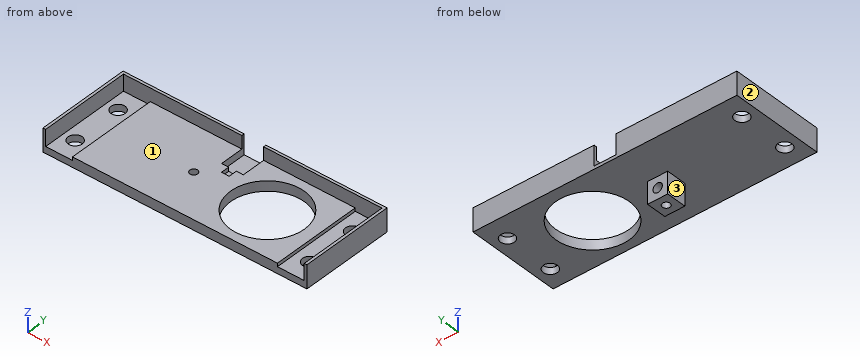
```python
from build123d import *

# Parameters (mm, degrees)
SKETCH_W        = 78.8
SKETCH_H        = 28
PAD_DEPTH       = 3
SKETCH001_R     = 11
POCKET_DEPTH    = 3.9
SKETCH002_W     = 0.8
SKETCH002_H     = 28
PAD001_DEPTH    = 3.9
SKETCH003_W     = 77.2
SKETCH003_H     = 0.8
PAD002_DEPTH    = 3.9
SKETCH004_W     = 8
SKETCH004_H     = 27.2
POCKET001_DEPTH = 1
SKETCH005_R     = 2.1
POCKET002_DEPTH = 5
SKETCH006_W     = 6
SKETCH006_H     = 6
PAD003_DEPTH    = 6.5
SKETCH007_R     = 1.15
POCKET003_DEPTH = 10
SKETCH008_R     = 1.4
POCKET004_DEPTH = 6
SKETCH009_W     = 2.3
SKETCH009_H     = 2.5
POCKET005_DEPTH = 1.2
SKETCH011_W     = 6.5
SKETCH011_H     = 8
POCKET006_DEPTH = 6


with BuildPart() as part:
    # Sketch → Pad (new body)
    with BuildSketch(Plane.XY):
        with Locations((0, 0.4)):
            Rectangle(SKETCH_W, SKETCH_H)
    extrude(amount=PAD_DEPTH)

    # Sketch001 (on Face6 of Pad) → Pocket (cut)
    with BuildSketch(Plane.XY.offset(3)):
        with Locations((16, 0)):
            Circle(SKETCH001_R)
    extrude(amount=-POCKET_DEPTH, mode=Mode.SUBTRACT)

    # Sketch002 (on Face5 of Pocket) → Pad001 (join)
    with BuildSketch(Plane.XY.offset(3)):
        with Locations((39, 0.4)):
            Rectangle(SKETCH002_W, SKETCH002_H)
        with Locations((-39, 0.4)):
            Rectangle(SKETCH002_W, SKETCH002_H)
    extrude(amount=PAD001_DEPTH)

    # Sketch003 (on Face6 of Pad001) → Pad002 (join)
    with BuildSketch(Plane.XY.offset(3)):
        with Locations((0, 14)):
            Rectangle(SKETCH003_W, SKETCH003_H)
    extrude(amount=PAD002_DEPTH)

    # Sketch004 (on Face16 of Pad002) → Pocket001 (cut)
    with BuildSketch(Plane.XY.offset(3)):
        with Locations((34.6, 0)):
            Rectangle(SKETCH004_W, SKETCH004_H)
        with Locations((-34.6, 0)):
            Rectangle(SKETCH004_W, SKETCH004_H)
    extrude(amount=-POCKET001_DEPTH, mode=Mode.SUBTRACT)

    # Sketch005 (on Face19 of Pocket001) → Pocket002 (cut)
    with BuildSketch(Plane.XY.offset(3)):
        with Locations((35, 7.5)):
            Circle(SKETCH005_R)
        with Locations((35, -7.5)):
            Circle(SKETCH005_R)
        with Locations((-35, 7.5)):
            Circle(SKETCH005_R)
        with Locations((-35, -7.5)):
            Circle(SKETCH005_R)
    extrude(amount=-POCKET002_DEPTH, mode=Mode.SUBTRACT)

    # Sketch006 (on Face4 of Pocket002) → Pad003 (join)
    with BuildSketch(Plane(origin=(0, 0, 0), x_dir=(1, 0, 0), z_dir=(0, 0, -1))):
        with Locations((-6, 0)):
            Rectangle(SKETCH006_W, SKETCH006_H)
    extrude(amount=PAD003_DEPTH)

    # Sketch007 (on Face32 of Pad003) → Pocket003 (cut)
    with BuildSketch(Plane(origin=(0, 0, -6.5), x_dir=(1, 0, 0), z_dir=(0, 0, -1))):
        with Locations((-6, 0)):
            Circle(SKETCH007_R)
    extrude(amount=-POCKET003_DEPTH, mode=Mode.SUBTRACT)

    # Sketch008 (on Face15 of Pocket003) → Pocket004 (cut)
    with BuildSketch(Plane.XZ.offset(3)):
        with Locations((-6, -3.25)):
            Circle(SKETCH008_R)
    extrude(amount=-POCKET004_DEPTH, mode=Mode.SUBTRACT)

    # Sketch009 (on Face27 of Pocket004) → Pocket005 (cut)
    with BuildSketch(Plane.XY.offset(3)):
        with Locations((0, 5.25)):
            Rectangle(SKETCH009_W, SKETCH009_H)
    extrude(amount=-POCKET005_DEPTH, mode=Mode.SUBTRACT)

    # Sketch011 (on Face21 of Pocket005) → Pocket006 (cut)
    with BuildSketch(Plane.XY.offset(6.9)):
        with Locations((0, 10.5)):
            Rectangle(SKETCH011_W, SKETCH011_H)
    extrude(amount=-POCKET006_DEPTH, mode=Mode.SUBTRACT)


solid = part.part
```
Can you work these out from the model? Positions are in its coordinate system, mm. Face numbers are marked on the shaded views. A direction names the side the tool comes from. Round coordinates to 2 decimals unless told otherwise and drop trailing zeros. Loops run counter-clockwise (first coordinate to the right, second up) from the corner with the lowest first, then second, coordinate; pieces in that order, holes last. Notation, with made-up numbers: (34, 56) -> (47, 56) arc R20 cw to (47, 92) -> close; hole circle Ø2 at (49, 86.5). An arc over 180 degrees is marked (long way). One line per item, written item: value. Start each with the question number.
1. If we section it at C-C, the plane z = -3.25: Write out the boundary of the cut face in (x, y), then the cut area to 3 significant figures.
2. For pin 1 (6.5 mm diameter, centred on y = 0.5, z = -4.5, fed in from +X); pin 2 (7 mm diameter, centred on x = 1, y = 10, fed in from +Z); pin 3 (1.5 mm diameter, centred on x = -27.5, y = -2, fed in from -Z), each with a flat end and sliding along its axis, tell me the tip position at first contact or that it passes through.
3. If we section it at A-A, the plane x = 16: Write out the boundary of the cut face in (y, z).
4. If we section it at B-B, the plane y = -6.5: Write out the boundary of the cut face in (x, z), then the cut area to 3 significant figures.
5. For the marked faces 1, 2 and 3, which set-ups out of +Z, -Z, +X, -X, +Y, -Y let a thin tool reach every point of the face, with its end or its side?
6. If we section it at D-D, the plane x = -35: Write out the boundary of the cut face in (y, z).
7. If I drill on probe 1 along X at (y, z) = (4.5, 5.75); probe 2 along Y at (x, z) = (16, 2.1); probe 3 along Z at (x, y) = (-6, 1.5), over which ranges is the centre line in solid material (lowest first)?
Calculated:
1. outline: (-9, -3) -> (-7.4, -3) -> (-7.4, 3) -> (-9, 3) -> close; (-4.6, -3) -> (-3, -3) -> (-3, 3) -> (-4.6, 3) -> close
1. area: 19.2 mm²
2. pin 1: stops at x = -3
2. pin 2: stops at z = 3
2. pin 3: stops at z = 0
3. outline: (-13.6, 0) -> (-11, 0) -> (-11, 3) -> (-13.6, 3) -> close; (11, 0) -> (14.4, 0) -> (14.4, 6.9) -> (13.6, 6.9) -> (13.6, 3) -> (11, 3) -> close
4. outline: (-39.4, 0) -> (-36.85, 0) -> (-36.85, 2) -> (-38.6, 2) -> (-38.6, 6.9) -> (-39.4, 6.9) -> close; (-33.15, 0) -> (7.13, 0) -> (7.13, 3) -> (-30.6, 3) -> (-30.6, 2) -> (-33.15, 2) -> close; (24.87, 0) -> (33.15, 0) -> (33.15, 2) -> (30.6, 2) -> (30.6, 3) -> (24.87, 3) -> close; (36.85, 0) -> (39.4, 0) -> (39.4, 6.9) -> (38.6, 6.9) -> (38.6, 2) -> (36.85, 2) -> close
4. area: 159 mm²
5. face 1: +Z, -Y
5. face 2: +Z, -Z, -X, +Y, -Y
5. face 3: -Z, -X, +Y, -Y
6. outline: (-13.6, 0) -> (-9.6, 0) -> (-9.6, 2) -> (-13.6, 2) -> close; (-5.4, 0) -> (5.4, 0) -> (5.4, 2) -> (-5.4, 2) -> close; (9.6, 0) -> (14.4, 0) -> (14.4, 6.9) -> (13.6, 6.9) -> (13.6, 2) -> (9.6, 2) -> close
7. probe 1: x = -39.4 to -38.6, 38.6 to 39.4
7. probe 2: y = -13.6 to -11, 11 to 14.4
7. probe 3: z = -6.5 to -4.65, -1.85 to 3
